from build123d import *

# Parameters (mm, degrees)
SCHIZZO1_R                   = 0.9
ESTRUSIONE_ESTRUSIONE1_DEPTH = 1
RACCORDO2_R                  = 0.5
SMUSSO2_SIZE                 = 0.05


with BuildPart() as part:
    # Schizzo1 → Estrusione-Estrusione1 (new body)
    with BuildSketch(Plane.XY):
        with BuildLine():
            Line((5.162187927, 7.372368399), (7.456493673, 10.648976576))
            ThreePointArc((7.456493673, 10.648976576), (0, -13), (-7.456493673, 10.648976576))
            Line((-7.456493673, 10.648976576), (-5.162187927, 7.372368399))
            ThreePointArc((-5.162187927, 7.372368399), (-6.363961031, 6.363961031), (-7.372368399, 5.162187927))
            Line((-7.372368399, 5.162187927), (-8.191520443, 5.735764364))
            ThreePointArc((-8.191520443, 5.735764364), (0, -10), (8.191520443, 5.735764364))
            Line((8.191520443, 5.735764364), (7.372368399, 5.162187927))
            ThreePointArc((7.372368399, 5.162187927), (6.363961031, 6.363961031), (5.162187927, 7.372368399))
        make_face()
        with Locations((-7.250430621, 7.373218425)):
            Circle(SCHIZZO1_R, mode=Mode.SUBTRACT)
        with Locations(Location((7.250430621, 7.373218425, 0), (0, 0, 180))):
            Circle(SCHIZZO1_R, mode=Mode.SUBTRACT)
    extrude(amount=ESTRUSIONE_ESTRUSIONE1_DEPTH)

    # Raccordo2
    raccordo2_edges = [part.edges().sort_by_distance(p)[0] for p in [
        (5.162187927, 7.372368399, 0.5),
        (7.372368399, 5.162187927, 0.5),
        (8.191520443, 5.735764364, 0.5),
        (-5.162187927, 7.372368399, 0.5),
        (-7.372368399, 5.162187927, 0.5),
        (-8.191520443, 5.735764364, 0.5),
    ]]
    fillet(raccordo2_edges, radius=RACCORDO2_R - 0.0001)  # a hair under: the kernel refuses the full size

    # Smusso2
    smusso2_edges = [part.edges().sort_by_distance(p)[0] for p in [
        (0, -13, 1),
        (6.448931556, 9.210028747, 1),
        (7.456493673, 10.648976576, 0.5),
        (-7.456493673, 10.648976576, 0.5),
        (-8.150430621, 7.373218425, 0),
        (-8.150430621, 7.373218425, 1),
        (8.150430621, 7.373218425, 0),
        (8.150430621, 7.373218425, 1),
        (6.363961031, 6.363961031, 0),
        (6.363961031, 6.363961031, 1),
        (-6.363961031, 6.363961031, 0),
        (0, -10, 0),
        (-6.448931556, 9.210028747, 0),
        (-7.410530845, 5.356443953, 0),
        (-5.356443953, 7.410530845, 0),
        (7.410530845, 5.356443953, 0),
        (5.356443953, 7.410530845, 0),
        (-6.363961031, 6.363961031, 1),
        (-6.448931556, 9.210028747, 1),
        (0, -10, 1),
        (-7.410530845, 5.356443953, 1),
        (-5.356443953, 7.410530845, 1),
        (7.410530845, 5.356443953, 1),
        (5.356443953, 7.410530845, 1),
        (8.157709655, 5.521840362, 0),
        (8.157709655, 5.521840362, 1),
        (-8.157709655, 5.521840362, 0),
        (-8.157709655, 5.521840362, 1),
        (6.448931556, 9.210028747, 0),
        (0, -13, 0),
    ]]
    chamfer(smusso2_edges, length=SMUSSO2_SIZE)


solid = part.part
Verification items for the finished model (mm, model axes). A direction names the side the tool comes from. Give positions to 0.01 mm unless a question says otherwise; leave off trailing zeros. Order: outer loops, then holes, each group sorted by start corner. A loop starts at its lowest first (then second) coordinate and runs counter-clockwise, first axis right, second up. Notation, with made-up numbers: M 0,-20 L 9,-20 A26 cw 9,14 Z; hole C 22.5,-20 d5. An arc over 180 degrees is marked long. Answer as a JSON object with one key per item and string values. Group by question number.
1) Scan lines: line 1 along X through (y, z) = (0, 0.35); line 2 along Y through (x, z) = (-6.5, 0.1); line 3 along X through (y, z) = (8, 0.4). Record each from-to range of solid material in increasing order. Write a range as [from, to].
2) Cross-section at A-A (y = 0). Enter the section's corners in (x, z), then the cut area to 3 significant figures.
3) Access from +Z, -Z, +X, -X, +Y, -Y to the whole of each face (thin tool, end or side, straight path). Record for faces 5 (the face through (-6.353, 6.375, 0.494)), 6 (the face through (-3, -10, 1)).
4) Cross-section at C-C (z = 0.5). Give the number of separate pieces and of enclosed holes in the cut face, then the cut area to 3 significant figures.
5) Cross-section at B-B (x = 0). Enter the section's corners in (y, z), then the cut area to 4 significant figures.
6) Mould release check, pull along X, two halves, no side actions. Record for faces 1 (the face through (-3, -10, 0)), 2 (the face through (0.46, -12.99, 0.49)), 3 (the face through (6.375, 6.353, 0.494)), 4 (the face through (6.42, 9.17, 0.49)): released by +X, released by -X, zero draft, split by the parting line, or undercut.
Result sheet:
{
 "1": {"line 1": "x = [-13, -10], [10, 13]", "line 2": "y = [-11.26, -7.6], [6.22, 6.88], [7.87, 9.28]", "line 3": "x = [-10.25, -7.9], [-6.6, -5.6], [5.6, 6.6], [7.9, 10.25]"},
 "2": {"outline": "M -13,0.05 L -12.95,0 L -10.05,0 L -10,0.05 L -10,0.95 L -10.05,1 L -12.95,1 L -13,0.95 Z; M 10,0.05 L 10.05,0 L 12.95,0 L 13,0.05 L 13,0.95 L 12.95,1 L 10.05,1 L 10,0.95 Z", "area": "5.99 mm2"},
 "3": {"face 5": "+Z, -Z", "face 6": "+Z, +X, -X, +Y, -Y"},
 "4": {"separate pieces": "1", "enclosed holes": "2", "area": "176 mm2"},
 "5": {"outline": "M -13,0.05 L -12.95,0 L -10.05,0 L -10,0.05 L -10,0.95 L -10.05,1 L -12.95,1 L -13,0.95 Z", "area": "2.995 mm2"},
 "6": {"face 1": "zero draft", "face 2": "split by the parting line", "face 3": "undercut", "face 4": "undercut"}
}
